from build123d import *

# Parameters (mm, degrees)
BOSS_EXTRUDE1_DEPTH            = 15
FILLET1_R                      = 2
M3_CLEARANCE_HOLE1_D           = 3.4
M3_CLEARANCE_HOLE1_ON_FACE_2_D = 3.4
SKETCH3_R                      = 3
CUT_EXTRUDE1_DEPTH             = 8
SKETCH4_R                      = 3
CUT_EXTRUDE2_DEPTH             = 8


with BuildPart() as part:
    # Sketch1 → Boss-Extrude1 (new body, symmetric)
    with BuildSketch(Plane(origin=(0, 0, 0), x_dir=(1, 0, 0), z_dir=(0, 1, 0))):
        Polygon((0, 0), (0, 32), (-10, 32), (-10, -10), (23, -10), (23, 0), align=None)
        Polygon((-8, 30), (-2, 30), (-2, 0.828427125), (-8, -5.171572875), align=None, mode=Mode.SUBTRACT)
        Polygon((21, -8), (-5.171572875, -8), (0.828427125, -2), (21, -2), align=None, mode=Mode.SUBTRACT)
    extrude(amount=BOSS_EXTRUDE1_DEPTH, both=True)

    # Fillet1
    fillet1_edges = [part.edges().sort_by_distance(p)[0] for p in [
        (-10, 0, 10),
        (-10, 0, -32),
        (21, 0, 8),
        (-8, 0, -30),
    ]]
    fillet(fillet1_edges, radius=FILLET1_R)

    # M3 Clearance Hole1 (through all)
    with Locations(Plane(origin=(15, -10, 0), x_dir=(-1, 0, 0), z_dir=(0, 0, -1))):
        with Locations((0, 0), (0, 20)):
            Hole(M3_CLEARANCE_HOLE1_D / 2)

    # M3 Clearance Hole1 on face 2 (through all)
    with Locations(Plane(origin=(0, 10, -24), x_dir=(0, 0, 1), z_dir=(1, 0, 0))):
        with Locations((0, 0), (0, 20)):
            Hole(M3_CLEARANCE_HOLE1_ON_FACE_2_D / 2)

    # Sketch3 → Cut-Extrude1 (cut)
    with BuildSketch(Plane.ZY.offset(10)):
        with Locations((-24, 10)):
            Circle(SKETCH3_R)
        with Locations((-24, -10)):
            Circle(SKETCH3_R)
    extrude(amount=-CUT_EXTRUDE1_DEPTH, mode=Mode.SUBTRACT)

    # Sketch4 → Cut-Extrude2 (cut)
    with BuildSketch(Plane.XY.offset(10)):
        with Locations((15, 10)):
            Circle(SKETCH4_R)
        with Locations((15, -10)):
            Circle(SKETCH4_R)
    extrude(amount=-CUT_EXTRUDE2_DEPTH, mode=Mode.SUBTRACT)


solid = part.part
For this review, take the finished solid that the model builds, in its own axes (mm). A direction names the side the tool comes from. Give positions to 0.01 mm unless a question says otherwise; leave off trailing zeros. Loops run counter-clockwise (first coordinate to the right, second up) from the corner with the lowest first, then second, coordinate; pieces in that order, holes last. Notation, with made-up numbers: (44, 33.5) -> (91, 33.5) arc R31 cw to (91, 67.5) -> close; hole circle Ø6 at (-3, 50). An arc over 180 degrees is marked (long way). One line per question, with ' | ' between items.
1) We need section D-D (x = 15). Write out the cut boundary in (y, z).
Resolved:
outline: (-15, 0) -> (-11.7, 0) -> (-11.7, 2) -> (-15, 2) -> close; (-15, 8) -> (-13, 8) -> (-13, 10) -> (-15, 10) -> close; (-8.3, 0) -> (8.3, 0) -> (8.3, 2) -> (-8.3, 2) -> close; (-7, 8) -> (7, 8) -> (7, 10) -> (-7, 10) -> close; (11.7, 0) -> (15, 0) -> (15, 2) -> (11.7, 2) -> close; (13, 8) -> (15, 8) -> (15, 10) -> (13, 10) -> close
2) For faces 1 (the cylindrical face through (-1.01, 10.65, -25.57)), 2 (the cylindrical face through (12.6, 8.2, 9)), 3 (the flat face through (-4.96, 0.21, 2.13)), 4 (the cylindrical face through (-9, -10, -27)), 5 (the flat face through (12, 0, 0)), list the 3-axis set-ups (+Z, -Z, +X, -X, +Y, -Y) from which the entire face can be reached by the end or side of a thin tool; tool diameter is ignored.
Resolved:
face 1: +X, -X | face 2: +Z | face 3: +Y, -Y | face 4: -X | face 5: -Z, +X, +Y, -Y
3) The part is to be moulded in two halves that separate along X. For faces 6 (the flat face through (-4, 0, -30)), 7 (the flat face through (7, 0, 10)), 8 (the cylindrical face through (-9.43, 0.21, -31.4)), 9 (the flat face through (0, 0, -16)), say which applies: +X half, -X half, draft (parallel to the pull), parting line (faces both ways), or undercut.
Resolved:
face 6: undercut | face 7: draft | face 8: -X half | face 9: +X half
4) We need section B-B (x = 10). Write out the cut boundary in (y, z).
Resolved:
outline: (-15, 0) -> (15, 0) -> (15, 2) -> (-15, 2) -> close; (-15, 8) -> (15, 8) -> (15, 10) -> (-15, 10) -> close
5) To check wall thickness, follow probe 1 along Y at (x, z) = (-1.1, -24); probe 2 along Y at (x, z) = (15, 9.05); probe 3 along X at (y, z) = (-2.5, -11.5). State the ranges of each line that lie inside material, in increasing order.
Resolved:
probe 1: y = -15 to -11.7, -8.3 to 8.3, 11.7 to 15 | probe 2: y = -15 to -13, -7 to 7, 13 to 15 | probe 3: x = -10 to -8, -2 to 0
6) We need section A-A (z = -6). Write out the cut boundary in (x, y), plus the area to 3 significant figures.
Resolved:
outline: (-10, -15) -> (-8, -15) -> (-8, 15) -> (-10, 15) -> close; (-2, -15) -> (0, -15) -> (0, 15) -> (-2, 15) -> close | area: 120 mm2
7) Insertion check: pin 1 Ø5 at (x, y) = (19.5, -6.5) entering from -Z; pin 2 Ø8 at (y, z) = (-0.5, -27.5) entering from +X; pin 3 Ø5 at (y, z) = (10, -24) entering from -X. Each pin has a flat end and moves straight along its axis. Give the tip position at first contact, or say it passes through.
Resolved:
pin 1: stops at z = 0 | pin 2: stops at x = 0 | pin 3: stops at x = -2
8) We need section C-C (y = -3.25). Write out the cut boundary in (x, z).
Resolved:
outline: (-10, -30) arc R2 ccw to (-8, -32) -> (0, -32) -> (0, 0) -> (23, 0) -> (23, 10) -> (-8, 10) arc R2 ccw to (-10, 8) -> close; hole (-8, -28) arc R2 ccw to (-6, -30) -> (-2, -30) -> (-2, -0.83) -> (-8, 5.17) -> close; hole (-5.17, 8) -> (0.83, 2) -> (21, 2) -> (21, 6) arc R2 ccw to (19, 8) -> close
